Geometry check sheet. Reference: the model listing, model coordinates, mm. A direction names the side the tool comes from. Give positions to 0.01 mm unless a question says otherwise; leave off trailing zeros. Order: outer loops, then holes, each group sorted by start corner. A loop starts at its lowest first (then second) coordinate and runs counter-clockwise, first axis right, second up.
```python
from build123d import *

# Parameters (mm, degrees)
SKETCH1_W           = 30
SKETCH1_H           = 40
SKETCH1_R           = 1.75
BOSS_EXTRUDE2_DEPTH = 3
SKETCH2_W           = 30
SKETCH2_H           = 20
BOSS_EXTRUDE3_DEPTH = 30
SKETCH3_R           = 6
CUT_EXTRUDE1_DEPTH  = 30


with BuildPart() as part:
    # Sketch1 → Boss-Extrude2 (new body)
    with BuildSketch(Plane(origin=(0, 0, 0), x_dir=(1, 0, 0), z_dir=(0, 1, 0))):
        Rectangle(SKETCH1_W, SKETCH1_H)
        with Locations(Location((-10, 15, 0), (0, 0, 270))):
            Circle(SKETCH1_R, mode=Mode.SUBTRACT)
        with Locations(Location((10, 15, 0), (0, 0, 270))):
            Circle(SKETCH1_R, mode=Mode.SUBTRACT)
        with Locations(Location((10, -15, 0), (0, 0, 270))):
            Circle(SKETCH1_R, mode=Mode.SUBTRACT)
        with Locations(Location((-10, -15, 0), (0, 0, 270))):
            Circle(SKETCH1_R, mode=Mode.SUBTRACT)
    extrude(amount=BOSS_EXTRUDE2_DEPTH)

    # Sketch2 → Boss-Extrude3 (add)
    with BuildSketch(Plane(origin=(0, 3, 0), x_dir=(1, 0, 0), z_dir=(0, 1, 0))):
        Rectangle(SKETCH2_W, SKETCH2_H)
    extrude(amount=BOSS_EXTRUDE3_DEPTH)

    # Sketch3 → Cut-Extrude1 (cut)
    with BuildSketch(Plane.ZY.offset(15)):
        with Locations((0, 23)):
            Circle(SKETCH3_R)
    extrude(amount=-CUT_EXTRUDE1_DEPTH, mode=Mode.SUBTRACT)


solid = part.part
```
Q1. Cross-section at C-C, the plane z = 0. Record the boundary of the cut face in (x, y).
Q2. Access from +Z, -Z, +X, -X, +Y, -Y to the whole of each face (thin tool, end or side, straight path). Record for faces 4 (the face through (0, 1, -20)), 5 (the face through (0, 3, -15)), 6 (the face through (0, 3, 15)).
Q3. Cross-section at D-D, the plane x = 4.5. Record the boundary of the cut face in (y, z).
Q4. Gauge pin test, flat ends, axial feed: P1, Ø9, axis at x = 3, y = 18.5, coming from the -Z side; P2, Ø11, axis at y = 23, z = 0, coming from the -X side; P3, Ø5, axis at x = 7.5, y = 19, coming from the +Z side; P4, Ø5, axis at x = -2.5, z = -13, coming from the +Y side. Record the tip position at first contact, or that the pin passes through.
Q5. Cross-section at B-B, the plane y = 23. Record the boundary of the cut face in (x, z), and give its area (3 significant figures).
Q6. Thickness scan on L1, parallel to X at y = 1, z = -15; L2, parallel to Z at x = -10.5, y = 13; L3, parallel to Y at x = 2.5, z = 0. Record the ranges inside material, lowest first.
Q7. Cross-section at A-A, the plane x = 10. Record the boundary of the cut face in (y, z).
Q8. Release check for a two-part mould opening along Z. For faces 1 (the face through (0, 33, 0)), 2 (the face through (11.5, 1.5, 15.9)), 3 (the face through (0, 18, 10)) record: pulls with the +Z half, pulls with the -Z half, needs draft (parallel to the pull), parting line crosses it, or undercut.
Answers follow:
1. outline: (-15, 0) - (15, 0) - (15, 17) - (-15, 17) - close; (-15, 29) - (15, 29) - (15, 33) - (-15, 33) - close
2. face 4: -Z, +X, -X, +Y, -Y
2. face 5: -Z, +X, -X, +Y
2. face 6: +Z, +X, -X, +Y
3. outline: (0, -20) - (3, -20) - (3, -10) - (33, -10) - (33, 10) - (3, 10) - (3, 20) - (0, 20) - close; hole circle Ø12 at (23, 0)
4. P1: stops at z = -10
4. P2: passes through
4. P3: stops at z = 10
4. P4: stops at y = 3
5. outline: (-15, -10) - (15, -10) - (15, -6) - (-15, -6) - close; (-15, 6) - (15, 6) - (15, 10) - (-15, 10) - close
5. area: 240 mm2
6. L1: x = -15 to -11.75, -8.25 to 8.25, 11.75 to 15
6. L2: z = -10 to 10
6. L3: y = 0 to 17, 29 to 33
7. outline: (0, -20) - (3, -20) - (3, -16.75) - (0, -16.75) - close; (0, -13.25) - (3, -13.25) - (3, -10) - (33, -10) - (33, 10) - (3, 10) - (3, 13.25) - (0, 13.25) - close; (0, 16.75) - (3, 16.75) - (3, 20) - (0, 20) - close; hole circle Ø12 at (23, 0)
8. face 1: needs draft
8. face 2: undercut
8. face 3: pulls with the +Z half
